from build123d import *

# Parameters (mm, degrees)
FILLET1_R       = 0.1
FILLET2_R       = 0.3
HEX_2_DEPTH     = 1.3
THDSCHPAT_COUNT = 21
THDSCHPAT_PITCH = 0.5


with BuildPart() as part:
    # BodySke → Base-Revolve (revolve)
    with BuildSketch(Plane.XY, mode=Mode.PRIVATE) as base_revolve_sk:
        Polygon((0, 0), (0, 2.75), (3, 2.75), (3, 1.5), (14.7195, 1.5), (15, 1.2195), (15, 0), align=None)
    revolve(base_revolve_sk.sketch.rotate(Axis((-31.75, 0, 0), (1, 0, 0)), 90), axis=Axis((-31.75, 0, 0), (1, 0, 0)))  # turned: the seam where the file's is

    # Fillet1
    fillet1_edges = [part.edges().sort_by_distance(p)[0] for p in [
        (3, 0, -1.5),
    ]]
    fillet(fillet1_edges, radius=FILLET1_R)

    # Fillet2
    fillet2_edges = [part.edges().sort_by_distance(p)[0] for p in [
        (0, 0, -2.75),
    ]]
    fillet(fillet2_edges, radius=FILLET2_R)

    # Sketch2 → Hex-PreBroach (revolve, cut)
    with BuildSketch(Plane.XY, mode=Mode.PRIVATE) as hex_prebroach_sk:
        Polygon((0, 1.26), (1.3, 1.26), (2.027461339, 0), (0, 0), align=None)
    revolve(hex_prebroach_sk.sketch.rotate(Axis((0, 0, 0), (1, 0, 0)), 90), axis=Axis((0, 0, 0), (1, 0, 0)), mode=Mode.SUBTRACT)  # turned: the seam where the file's is

    # Sketch3 → Hex 2 (cut)
    with BuildSketch(Plane(origin=(0, 0, 0), x_dir=(0, 0.5, 0.866025404), z_dir=(-1, 0, 0))):
        Polygon((0.727461339, 1.26), (-0.727461339, 1.26), (-1.454922678, 0), (-0.727461339, -1.26), (0.727461339, -1.26), (1.454922678, 0), align=None)
    extrude(amount=-HEX_2_DEPTH, mode=Mode.SUBTRACT)

    # ThdSchSke → ThreadSchematic (revolve, cut)
    with BuildSketch(Plane.XY, mode=Mode.PRIVATE) as threadschematic_sk:
        Polygon((4.5, -1.2195), (4.303591786, -1.5), (4.303591786, -1.875), (4.696408214, -1.875), (4.696408214, -1.5), align=None)
    threadschematic = revolve(threadschematic_sk.sketch.rotate(Axis((-3.175, 0, 0), (1, 0, 0)), 270), axis=Axis((-3.175, 0, 0), (1, 0, 0)), mode=Mode.SUBTRACT)  # turned: the seam where the file's is

    # ThdSchPat: ThreadSchematic ×21
    with Locations(*[(i * THDSCHPAT_PITCH, 0, 0) for i in range(1, THDSCHPAT_COUNT)]):
        add(threadschematic, mode=Mode.SUBTRACT)


solid = part.part
Input: part model. Units: mm. Frame: model coordinates. Give positions to 0.01 mm unless a question says otherwise; leave off trailing zeros. Use one line per item in the form item = value.
1. First-contact query: pin 1 (2 mm diameter, centred on x = 7.5, z = 0.5, fed in from +Y); pin 2 (2 mm diameter, centred on x = 3, y = -2, fed in from +Z). Flat tips, straight axial feed; report the tip coordinate or a pass-through.
Numbers:
pin_1 = 1.5
pin_2 = 2.56
2. Line query: L1, parallel to Z at x = 1.25, y = 0.1; L2, parallel to X at y = 2.3, z = -0.7; L3, parallel to Y at x = 7.25, z = 0.1. Output: solid intervals per line, ascending.
Numbers:
L1 = -2.75 to -1.26, 1.26 to 2.75
L2 = 0 to 3
L3 = -1.5 to 1.5
3. Pull-direction query (Z, two-part tool) for faces 1 (the face through (3.71, -0.45, 1.43)), 2 (the face through (0.641, 1.096, -0.621)); classes: released by +Z, released by -Z, zero draft, split by the parting line, or undercut.
Numbers:
face_1 = split by the parting line
face_2 = undercut
